Verification items for this drawing (mm, ordinates from the low corner). A direction names the side the tool comes from. Round coordinates to 2 decimals unless told otherwise and drop trailing zeros. Order: outer loops, then holes, each group sorted by start corner. A loop starts at its lowest first (then second) coordinate and runs counter-clockwise, first axis right, second up. Notation, with made-up numbers: (19, 27.5) -> (45, 27.5) arc R35 ccw to (45, 63.5) -> close; hole circle Ø1 at (-36.5, 74). An arc over 180 degrees is marked (long way). Answer in a Markdown table with one row per item.
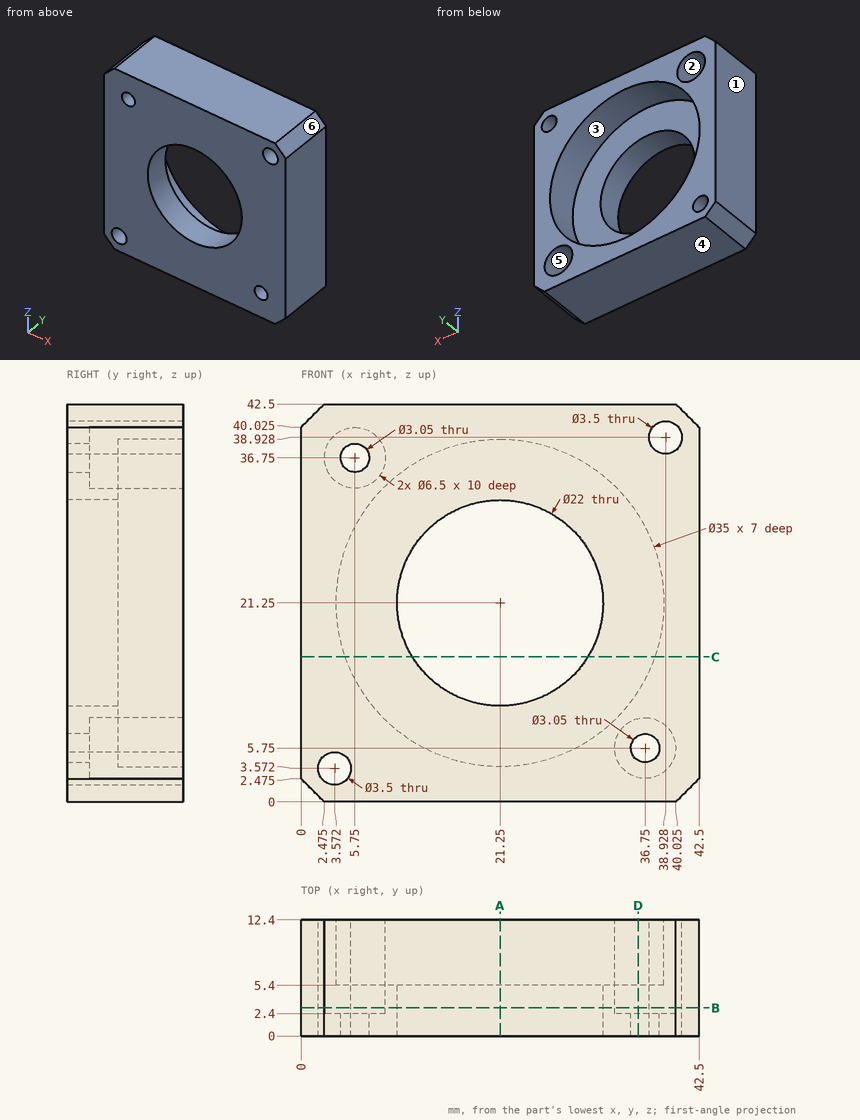
Item 1: Cross-section at C-C (z = 15.5). Record the boundary of the cut face in (x, y).
Result sheet:
| item | result |
|---|---|
| outline | (0, 0) -> (11.87, 0) -> (11.87, 5.4) -> (4.72, 5.4) -> (4.72, 12.4) -> (0, 12.4) -> close; (30.63, 0) -> (42.5, 0) -> (42.5, 12.4) -> (37.78, 12.4) -> (37.78, 5.4) -> (30.63, 5.4) -> close |
Item 2: Cross-section at B-B (y = 3). State how many separate pieces and enclosed holes the cut face has, and give its area (3 significant figures).
Result sheet:
| item | result |
|---|---|
| separate pieces | 1 |
| enclosed holes | 5 |
| area | 1,330 mm^2 |
Item 3: Set-up check for the marked faces 1 and 2: record each of +Z, -Z, +X, -X, +Y, -Y from which the full face is reachable in a straight line by a thin tool's end or side.
Result sheet:
| item | result |
|---|---|
| face 1 | +Z, -Z, -X, +Y, -Y |
| face 2 | +Y |
Item 4: Cross-section at A-A (x = 21.25). Record the boundary of the cut face in (y, z).
Result sheet:
| item | result |
|---|---|
| outline | (0, 0) -> (12.4, 0) -> (12.4, 3.75) -> (5.4, 3.75) -> (5.4, 10.25) -> (0, 10.25) -> close; (0, 32.25) -> (5.4, 32.25) -> (5.4, 38.75) -> (12.4, 38.75) -> (12.4, 42.5) -> (0, 42.5) -> close |
Item 5: Cross-section at D-D (x = 36). Record the boundary of the cut face in (y, z).
Result sheet:
| item | result |
|---|---|
| outline | (0, 0) -> (12.4, 0) -> (12.4, 2.59) -> (2.4, 2.59) -> (2.4, 4.42) -> (0, 4.42) -> close; (0, 7.08) -> (2.4, 7.08) -> (2.4, 8.91) -> (12.4, 8.91) -> (12.4, 11.83) -> (5.4, 11.83) -> (5.4, 30.67) -> (12.4, 30.67) -> (12.4, 42.5) -> (0, 42.5) -> close |
Item 6: Depth check by flat-ended pin: P1, Ø5, axis at x = 5.75, z = 36.75, coming from the +Y side; P2, Ø7, axis at x = 37, z = 5, coming from the +Y side; P3, Ø8, axis at x = 19, z = 12.5, coming from the +Y side. Enter the tip coordinate at first touch or a pass-through.
Result sheet:
| item | result |
|---|---|
| P1 | stops at y = 2.4 |
| P2 | stops at y = 12.4 |
| P3 | stops at y = 5.4 |
Item 7: Mould release check, pull along X, two halves, no side actions. Record for the marked faces 3, 4, 5 and 6: pulls with the +X half, pulls with the -X half, needs draft (parallel to the pull), parting line crosses it, or undercut.
Result sheet:
| item | result |
|---|---|
| face 3 | undercut |
| face 4 | needs draft |
| face 5 | undercut |
| face 6 | pulls with the +X half |
Item 8: Scan lines: line 1 (Z direction, x = 6, y = 5); line 2 (X direction, y = 1, z = 5.75) (1 decimal). Record each from-to range of solid material in increasing order. Write a range as [from, to].
Result sheet:
| item | result |
|---|---|
| line 1 | z = [0, 33.51], [39.99, 42.5] |
| line 2 | x = [0, 35.2], [38.3, 42.5] |
